```python
from build123d import *

# Parameters (mm, degrees)
SKETCH1_W           = 150
SKETCH1_H           = 150
SKETCH1_R           = 1.5
SKETCH1_W_2         = 85
SKETCH1_H_2         = 85
BOSS_EXTRUDE1_DEPTH = 8
SKETCH3_W           = 128
SKETCH3_H           = 128
CUT_EXTRUDE2_DEPTH  = 2.85
FILLET1_R           = 3
SKETCH4_R           = 2.5
CUT_EXTRUDE3_DEPTH  = 2.5
SKETCH5_R           = 1.75
CUT_EXTRUDE4_DEPTH  = 23


with BuildPart() as part:
    # Sketch1 → Boss-Extrude1 (new body)
    with BuildSketch(Plane.XY):
        Rectangle(SKETCH1_W, SKETCH1_H)
        with Locations((-50, 50)):
            Circle(SKETCH1_R, mode=Mode.SUBTRACT)
        with Locations((50, 50)):
            Circle(SKETCH1_R, mode=Mode.SUBTRACT)
        with Locations((50, -50)):
            Circle(SKETCH1_R, mode=Mode.SUBTRACT)
        with Locations((-50, -50)):
            Circle(SKETCH1_R, mode=Mode.SUBTRACT)
        Rectangle(SKETCH1_W_2, SKETCH1_H_2, mode=Mode.SUBTRACT)
    extrude(amount=BOSS_EXTRUDE1_DEPTH)

    # Sketch3 → Cut-Extrude2 (cut)
    with BuildSketch(Plane.XY.offset(8)):
        Rectangle(SKETCH3_W, SKETCH3_H)
    extrude(amount=-CUT_EXTRUDE2_DEPTH, mode=Mode.SUBTRACT)

    # Fillet1
    fillet1_edges = [part.edges().sort_by_distance(p)[0] for p in [
        (75, -75, 4),
        (-75, -75, 4),
        (-75, 75, 4),
        (75, 75, 4),
    ]]
    fillet(fillet1_edges, radius=FILLET1_R)

    # Sketch4 → Cut-Extrude3 (cut)
    with BuildSketch(Plane(origin=(0, 0, 5.15), x_dir=(-1, 0, 0), z_dir=(0, 0, -1))):
        with Locations((-50, 50)):
            Circle(SKETCH4_R)
        with Locations((50, 50)):
            Circle(SKETCH4_R)
        with Locations((50, -50)):
            Circle(SKETCH4_R)
        with Locations((-50, -50)):
            Circle(SKETCH4_R)
    extrude(amount=CUT_EXTRUDE3_DEPTH, mode=Mode.SUBTRACT)

    # Sketch5 → Cut-Extrude4 (cut)
    with BuildSketch(Plane.XY.offset(8)):
        with Locations((0, 69.431322576)):
            Circle(SKETCH5_R)
        with Locations((-69.610191061, 69.610191061)):
            Circle(SKETCH5_R)
        with Locations((69.431322576, 0)):
            Circle(SKETCH5_R)
        with Locations((69.610191061, 69.610191061)):
            Circle(SKETCH5_R)
        with Locations((0, -69.431322576)):
            Circle(SKETCH5_R)
        with Locations((69.610191061, -69.610191061)):
            Circle(SKETCH5_R)
        with Locations((-69.431322576, 0)):
            Circle(SKETCH5_R)
        with Locations((-69.610191061, -69.610191061)):
            Circle(SKETCH5_R)
    extrude(amount=-CUT_EXTRUDE4_DEPTH, mode=Mode.SUBTRACT)


solid = part.part
```
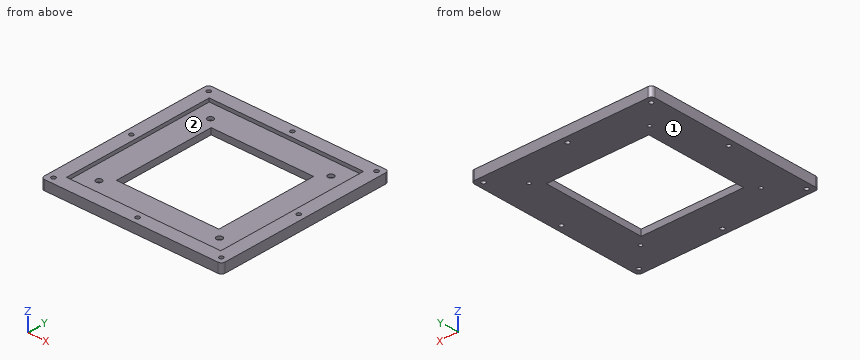
Geometry: final body of the model. Coordinates: model frame, mm. Face numbers are marked on the shaded views. A direction names the side the tool comes from. Round coordinates to 2 decimals unless told otherwise and drop trailing zeros. Write each loop counter-clockwise with the first axis right and the second up, starting at its lowest first coordinate (ties: lowest second). Pieces come first, ordered by that corner, then holes.
Item 1: Section query A-A (x = 0). Return loops of the section in (y, z).
Item 2: Section query D-D (z = 6.75). Give the number of separate pieces and of enclosed holes in the cut face, plus the area to 3 significant figures.
Item 3: Set-up query: the marked faces 1 and 2. Return all of +Z, -Z, +X, -X, +Y, -Y with unobstructed straight access to the full face (end or side cutting, diameter ignored); none if empty.
Item 4: Material intervals for L1, parallel to Y at x = -50, z = 4.15; L2, parallel to X at y = 50, z = 0.8; L3, parallel to Y at x = 21, z = 3, sorted ascending.
Item 5: Section query B-B (y = -27.5). Return loops of the section in (x, z), plus the area to 3 significant figures.
Item 6: Pin query (flat end, axial travel): P1, Ø4.5, axis at x = 0, y = -69.43, coming from the -Z side; P2, Ø4, axis at x = -50, y = -50, coming from the +Z side; P3, Ø8, axis at x = -38, y = 29, coming from the +Z side; P4, Ø5.5, axis at x = 49.5, y = -51, coming from the +Z side. Return the tip coordinate at first contact, or that it passes through.
Completed:
1. outline: (-75, 0) - (-71.18, 0) - (-71.18, 8) - (-75, 8) - close; (-67.68, 0) - (-42.5, 0) - (-42.5, 5.15) - (-64, 5.15) - (-64, 8) - (-67.68, 8) - close; (42.5, 0) - (67.68, 0) - (67.68, 8) - (64, 8) - (64, 5.15) - (42.5, 5.15) - close; (71.18, 0) - (75, 0) - (75, 8) - (71.18, 8) - close
2. separate pieces: 1
2. enclosed holes: 9
2. area: 6,030 mm2
3. face 1: -Z, +X, -X, +Y, -Y
3. face 2: +Z
4. L1: y = -75 to -52.5, -47.5 to 47.5, 52.5 to 75
4. L2: x = -75 to -51.5, -48.5 to 48.5, 51.5 to 75
4. L3: y = -75 to -42.5, 42.5 to 75
5. outline: (-75, 0) - (-42.5, 0) - (-42.5, 5.15) - (-64, 5.15) - (-64, 8) - (-75, 8) - close; (42.5, 0) - (75, 0) - (75, 8) - (64, 8) - (64, 5.15) - (42.5, 5.15) - close
5. area: 397 mm2
6. P1: stops at z = 0
6. P2: stops at z = 2.65
6. P3: passes through
6. P4: stops at z = 5.15
